Build history of the part. All positions in model axes, mm. Round coordinates to 2 decimals unless told otherwise and drop trailing zeros. Write each loop counter-clockwise with the first axis right and the second up, starting at its lowest first coordinate (ties: lowest second). Pieces come first, ordered by that corner, then holes. Notation, with made-up numbers: (-39, 2) -> (12, 2) arc R8 ccw to (12, 9) -> close; hole circle Ø3 at (86, 54.25). An arc over 180 degrees is marked (long way). Answer in a Markdown table with one row per item.
```python
from build123d import *

# Parameters (mm, degrees)
BOSS_EXTRUDE1_DEPTH     = 75
SKETCH2_R               = 3
CUT_EXTRUDE1_DEPTH      = 6
CUT_EXTRUDE1_DEPTH_BACK = 6


with BuildPart() as part:
    # Sketch1 → Boss-Extrude1 (new body, symmetric)
    with BuildSketch(Plane(origin=(0, 0, 0), x_dir=(0, 0, -1), z_dir=(1, 0, 0))):
        Polygon((0, 5.773502692), (-5, 2.886751346), (-5, -2.886751346), (0, -5.773502692), (5, -2.886751346), (5, 2.886751346), align=None)
    extrude(amount=BOSS_EXTRUDE1_DEPTH, both=True)

    # Sketch2 → Cut-Extrude1 (cut, two sides)
    with BuildSketch(Plane.XY) as cut_extrude1_sk:
        with Locations((65, 0)):
            Circle(SKETCH2_R)
        with Locations((-65, 0)):
            Circle(SKETCH2_R)
    extrude(amount=CUT_EXTRUDE1_DEPTH, mode=Mode.SUBTRACT)
    extrude(cut_extrude1_sk.sketch, amount=-CUT_EXTRUDE1_DEPTH_BACK, mode=Mode.SUBTRACT)


solid = part.part
```
Q1. Saw through at B-B on z = 3. Write the cut outline in (x, y), plus the area to 3 significant figures.
A:
| item | result |
|---|---|
| outline | (-75, -4.04) -> (75, -4.04) -> (75, 4.04) -> (-75, 4.04) -> close; hole circle Ø6 at (-65, 0); hole circle Ø6 at (65, 0) |
| area | 1,160 mm² |
Q2. Drop flat-ended pins along their axis: P1, Ø6, axis at x = 44.5, z = 2.5, coming from the +Y side; P2, Ø1, axis at x = 42.5, z = 1, coming from the -Y side; P3, Ø1.5, axis at x = 38.5, z = -3.5, coming from the -Y side. Give the stop position or say it passes through.
A:
| item | result |
|---|---|
| P1 | y = 5.77 |
| P2 | y = -5.48 |
| P3 | y = -4.19 |
Q3. Saw through at C-C on x = -38. Write the cut outline in (y, z), plus the area to 3 significant figures.
A:
| item | result |
|---|---|
| outline | (-5.77, 0) -> (-2.89, -5) -> (2.89, -5) -> (5.77, 0) -> (2.89, 5) -> (-2.89, 5) -> close |
| area | 86.6 mm² |
Q4. Wall check: line 1 (X direction, y = 0, z = -3.1); line 2 (X direction, y = 1.25, z = 3); line 3 (Y direction, x = 65, z = -1.75). Give the ranges that are in metal, low to high. Write a range as [from, to].
A:
| item | result |
|---|---|
| line 1 | [-75, -68], [-62, 62], [68, 75] |
| line 2 | [-75, -67.73], [-62.27, 62.27], [67.73, 75] |
| line 3 | [-4.76, -3], [3, 4.76] |
Q5. Saw through at D-D on z = -3.5. Write the cut outline in (x, y).
A:
| item | result |
|---|---|
| outline | (-75, -3.75) -> (75, -3.75) -> (75, 3.75) -> (-75, 3.75) -> close; hole circle Ø6 at (-65, 0); hole circle Ø6 at (65, 0) |
Q6. Saw through at A-A on y = 0. Write the cut outline in (x, z), plus the area to 3 significant figures.
A:
| item | result |
|---|---|
| outline | (-75, -5) -> (-68, -5) -> (-68, 5) -> (-75, 5) -> close; (-62, -5) -> (62, -5) -> (62, 5) -> (-62, 5) -> close; (68, -5) -> (75, -5) -> (75, 5) -> (68, 5) -> close |
| area | 1,380 mm² |
